Could you check a few things on this drawing? It's one solid part, dimensions in mm from its lowest x, y, z. Round coordinates to 2 decimals unless told otherwise and drop trailing zeros. Order: outer loops, then holes, each group sorted by start corner. A loop starts at its lowest first (then second) coordinate and runs counter-clockwise, first axis right, second up. Notation, with made-up numbers: (4, 40.25) -> (19, 40.25) arc R24 cw to (19, 70.25) -> close; hole circle Ø3 at (54.25, -32). An arc over 180 degrees is marked (long way). Use a Markdown table: item, result. Add a question column.
(1) If I drill on probe 1 along X at (y, z) = (33, 2.4) (1 decimal); probe 2 along X at (y, z) = (33.5, 4.75) (1 decimal); probe 3 along X at (y, z) = (18, 1.2), over which ranges is the centre line in solid material (lowest first)?
(2) I want a section at C-C, the plane x = 23.5. Please give me the cut outline in (y, z) (1 decimal).
(3) I want a section at A-A, the plane y = 33.5. Please give me the cut outline in (x, z).
(4) I'm going to push flat-ended pins straight in: P1, Ø3, axis at y = 23, z = 1, coming from the +X side; P2, Ø3, axis at x = 14.5, z = 3.5, coming from the -Y side; P3, Ø1.5, axis at y = 26, z = 3.5, coming from the +X side. Where does each tip first touch, or does it pass through?
(5) I want a section at D-D, the plane z = 1.05. Please give me the cut outline in (x, y).
(6) Thinking about a two-plate mould opening in Y: for the marked faces 1, 2 and 3, which applies, pulls with the +Y half, pulls with the -Y half, needs draft (parallel to the pull), parting line crosses it, or undercut?
(7) I want a section at B-B, the plane x = 29. Please give me the cut outline in (y, z), then the cut area to 3 significant figures.
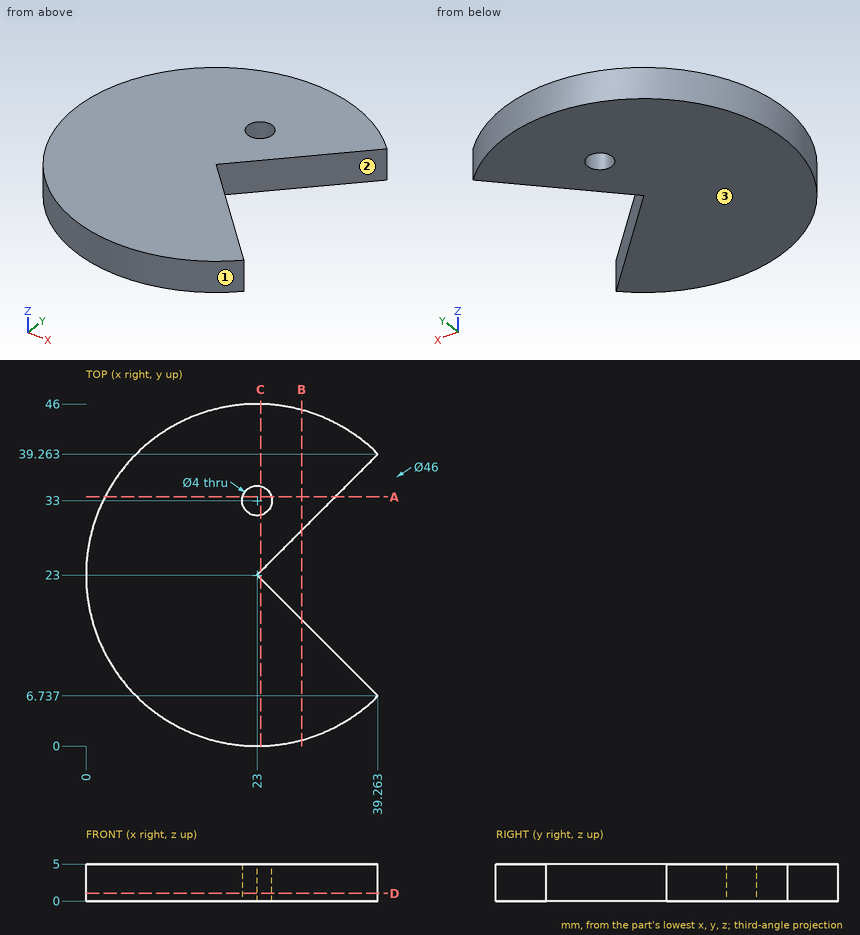
Taken from the geometry:
| question | item | result |
|---|---|---|
| 1 | probe 1 | x = 2.3 to 21, 25 to 33 |
| 1 | probe 2 | x = 2.5 to 21.1, 24.9 to 33.5 |
| 1 | probe 3 | x = 0.55 to 28 |
| 2 | outline | (0, 0) -> (22.5, 0) -> (22.5, 5) -> (0, 5) -> close; (23.5, 0) -> (31.1, 0) -> (31.1, 5) -> (23.5, 5) -> close; (34.9, 0) -> (46, 0) -> (46, 5) -> (34.9, 5) -> close |
| 3 | outline | (2.54, 0) -> (21.06, 0) -> (21.06, 5) -> (2.54, 5) -> close; (24.94, 0) -> (33.5, 0) -> (33.5, 5) -> (24.94, 5) -> close |
| 4 | P1 | stops at x = 24.5 |
| 4 | P2 | stops at y = 1.09 |
| 4 | P3 | stops at x = 26.75 |
| 5 | outline | (23, 23) -> (39.26, 39.26) arc R23 ccw (long way) to (39.26, 6.74) -> close; hole circle Ø4 at (23, 33) |
| 6 | face 1 | parting line crosses it |
| 6 | face 2 | undercut |
| 6 | face 3 | needs draft |
| 7 | outline | (0.8, 0) -> (17, 0) -> (17, 5) -> (0.8, 5) -> close; (29, 0) -> (45.2, 0) -> (45.2, 5) -> (29, 5) -> close |
| 7 | area | 162 mm2 |
